Can you work these out from the model? Positions are in its coordinate system, mm. A direction names the side the tool comes from. Give positions to 0.01 mm unless a question says otherwise; leave off trailing zeros. Order: outer loops, then holes, each group sorted by start corner. A loop starts at its lowest first (then second) coordinate and runs counter-clockwise, first axis right, second up. Notation, with made-up numbers: (-24.5, -5.75) - (26.5, -5.75) arc R28 cw to (26.5, 16.25) - close; hole circle Ø10 at (69.5, 83.25). An arc over 180 degrees is marked (long way). One line per question, with ' | ' between items.
Autodesk Inventor part; units mm, degrees
ref_plane "YZ Plane" through (0, 0, 0) normal (1, 0, 0) x (0, 1, 0)
ref_plane "XZ Plane" through (0, 0, 0) normal (0, 1, 0) x (-1, 0, 0)
ref_plane "XY Plane" through (0, 0, 0) normal (0, 0, 1) x (1, 0, 0)
sketch "Sketch1" plane through (0, 0, 0) normal (0, 0, 1) x (1, 0, 0)
  line L0 (-2.75, 1.59) -> (0, 3.18)
  line L1 (0, -3.18) -> (-2.75, -1.59)
  line L2 (-2.75, 1.59) -> (-2.75, -1.59)
  line L3 (2.75, 1.59) -> (0, 3.18)
  line L4 (0, -3.18) -> (2.75, -1.59)
  line L5 (2.75, 1.59) -> (2.75, -1.59)
  point P0 (0, 0)
extrude "Extrusion1" add sketch "Sketch1" along normal blind 19
sketch "Sketch2" plane through (0, 0, 19) normal (0, 0, 1) x (1, 0, 0)
  circle A0 centre (0, 0) radius 1.5
  dimension "d20" = 3
hole "Hole1" at (0, 0, 19) direction (0, 0, -1) diameter 2.459 depth 8.8 tip angle 118
fillet "Fillet1" radius 0.1 6 edges at (0, 3.18, 9.5) (2.75, 1.59, 9.5) (-2.75, 1.59, 9.5) (2.75, -1.59, 9.5) (0, -3.18, 9.5) (-2.75, -1.59, 9.5)
sketch "Sketch4" plane through (0, 0, 0) normal (0, 0, -1) x (-1, 0, 0)
  circle A0 centre (0, 0) radius 1.5
  dimension "d29" = 3
extrude "Extrusion2" add sketch "Sketch4" along normal blind 6.4
thread "Thread1"
fillet "Fillet2" radius 0.2 1 edges at (1.5, 0, -6.4)
properties part number "spacer" material "Steel, Mild"
(1) Imagine slicing it at A-A (z = 16.5). List the corners of the cut face in (x, y) for me.
Answer below:
outline: (-2.75, -1.53) arc R0.1 ccw to (-2.7, -1.62) - (-0.05, -3.15) arc R0.1 ccw to (0.05, -3.15) - (2.7, -1.62) arc R0.1 ccw to (2.75, -1.53) - (2.75, 1.53) arc R0.1 ccw to (2.7, 1.62) - (0.05, 3.15) arc R0.1 ccw to (-0.05, 3.15) - (-2.7, 1.62) arc R0.1 ccw to (-2.75, 1.53) - close; hole circle Ø2.46 at (0, 0)
(2) Will these pins go through, and if not, where does the flat tip stop? pin 1 (1 mm diameter, centred on x = -1, y = -1, fed in from -Z); pin 2 (1.5 mm diameter, centred on x = -1, z = 10.5, fed in from +Y); pin 3 (1 mm diameter, centred on x = -2, z = 5, fed in from -Y).
Answer below:
pin 1: z = -6.4 | pin 2: y = 3.04 | pin 3: y = -2.31
(3) On a 3-axis mill with a long thin cutter (end or side, diameter ignored), from which of +Z, -Z, +X, -X, +Y, -Y can I reach the whole of each face in a straight line? I mean faces 5 (the face through (0, -1.4, 19)), 6 (the face through (1.5, -0.07, -3.06)). Say none if no direction works.
Answer below:
face 5: +Z, +X, -X, +Y, -Y | face 6: -Z
(4) If I drill on line 1 (Y direction, x = 0, z = 14); line 2 (X direction, y = 0, z = 15); line 3 (X direction, y = 1, z = 16.25), over which ranges is the centre line in solid material (lowest first)?
Answer below:
line 1: -3.16 to -1.23, 1.23 to 3.16 | line 2: -2.75 to -1.23, 1.23 to 2.75 | line 3: -2.75 to -0.72, 0.72 to 2.75
(5) Imagine slicing it at C-C (x = -1.75). List the corners of the cut face in (y, z) for me.
Answer below:
outline: (-2.17, 0) - (2.17, 0) - (2.17, 19) - (-2.17, 19) - close
(6) Imagine slicing it at D-D (y = -2.5). List the corners of the cut face in (x, z) for me.
Answer below:
outline: (-1.18, 0) - (1.18, 0) - (1.18, 19) - (-1.18, 19) - close
(7) If we mould it in two halves opening along X, with no side actions, what happens to faces 1 (the face through (0.064, -0.204, 9.59)), 2 (the face through (-1.394, 2.374, 9.367)), 3 (the face through (-1.3, -1.4, 0)), 4 (the face through (0.748, 0.976, 14.538))? For each: released by +X, released by -X, zero draft, split by the parting line, or undercut.
Answer below:
face 1: undercut | face 2: released by -X | face 3: zero draft | face 4: undercut
(8) Imagine slicing it at B-B (z = 1.5). List the corners of the cut face in (x, y) for me, and give its area (3 significant figures).
Answer below:
outline: (-2.75, -1.53) arc R0.1 ccw to (-2.7, -1.62) - (-0.05, -3.15) arc R0.1 ccw to (0.05, -3.15) - (2.7, -1.62) arc R0.1 ccw to (2.75, -1.53) - (2.75, 1.53) arc R0.1 ccw to (2.7, 1.62) - (0.05, 3.15) arc R0.1 ccw to (-0.05, 3.15) - (-2.7, 1.62) arc R0.1 ccw to (-2.75, 1.53) - close | area: 26.2 mm^2
